The drawing under review shows one solid part. Ordinate dimensions are in mm from its lowest x, y, z. A direction names the side the tool comes from. Round coordinates to 2 decimals unless told otherwise and drop trailing zeros. Order: outer loops, then holes, each group sorted by start corner. A loop starts at its lowest first (then second) coordinate and runs counter-clockwise, first axis right, second up. Notation, with made-up numbers: (-14.75, -18) -> (2.25, -18) arc R27 cw to (2.25, 7) -> close; hole circle Ø11 at (-0.5, 12.5). An arc over 180 degrees is marked (long way). Return JSON: item names as keys, results as strings. Group by question number.
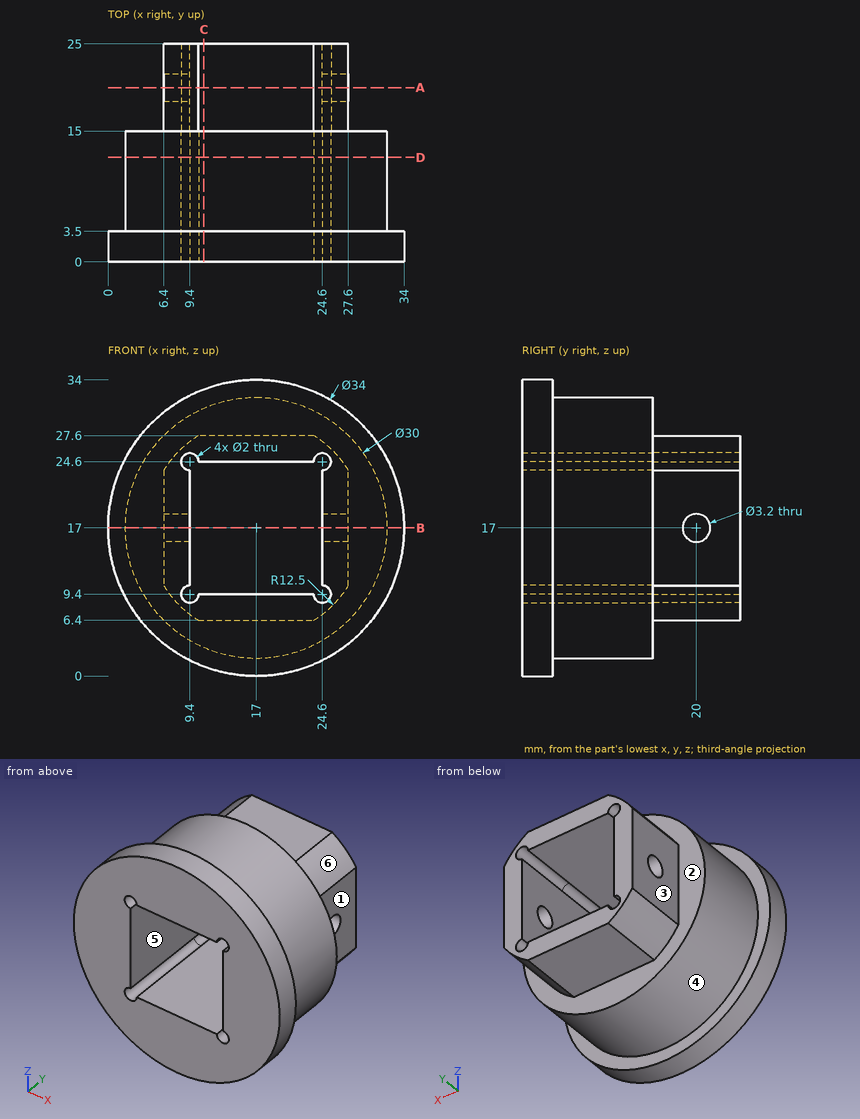
Item 1: Insertion check: pin 1 Ø5 at (y, z) = (18.5, 16) entering from -X; pin 2 Ø14.5 at (x, y) = (14, 16) entering from -Z; pin 3 Ø5 at (y, z) = (20, 17) entering from +X; pin 4 Ø8 at (x, z) = (26.5, 6.5) entering from -Y. Each pin has a flat end and moves straight along its axis. Give the tip position at first contact, or say it passes through.
Item 2: Consider section B-B on z = 17. State the section outline as (x, y) points, plus the area to 3 significant figures.
Item 3: Consider section A-A on y = 20. State the section outline as (x, z) points.
Item 4: Wall thickness on line 1 along X through (y, z) = (15.5, 19); line 2 along Y through (x, z) = (7.05, 17): over which ranges is each line inside the solid? List them lowest first.
Item 5: Consider section D-D on y = 12. State the section outline as (x, z) points, plus the area to 3 significant figures.
Item 6: Consider section C-C on x = 11. State the section outline as (y, z) points, plus the area to 3 significant figures.
Item 7: The part is to be moulded in two halves that separate along X. For the marked faces 4, 5 and 6, say which applies: +X half, -X half, draft (parallel to the pull), parting line (faces both ways), or undercut.
Item 8: For the marked faces 1, 2 and 3, list the 3-axis set-ups (+Z, -Z, +X, -X, +Y, -Y) from which the entire face can be reached by the end or side of a thin tool; tool diameter is ignored.
Values:
{
 "1": {"pin 1": "x = 6.4", "pin 2": "z = 2", "pin 3": "x = 27.6", "pin 4": "y = 0"},
 "2": {"outline": "(0, 0) -> (9.4, 0) -> (9.4, 18.4) -> (6.4, 18.4) -> (6.4, 15) -> (2, 15) -> (2, 3.5) -> (0, 3.5) -> close; (6.4, 21.6) -> (9.4, 21.6) -> (9.4, 25) -> (6.4, 25) -> close; (24.6, 0) -> (34, 0) -> (34, 3.5) -> (32, 3.5) -> (32, 15) -> (27.6, 15) -> (27.6, 18.4) -> (24.6, 18.4) -> close; (24.6, 21.6) -> (27.6, 21.6) -> (27.6, 25) -> (24.6, 25) -> close", "area": "277 mm^2"},
 "3": {"outline": "(6.4, 10.38) arc R12.5 ccw to (10.38, 6.4) -> (23.62, 6.4) arc R12.5 ccw to (27.6, 10.38) -> (27.6, 15.4) -> (24.6, 15.4) -> (24.6, 10.4) arc R1 cw (long way) to (23.6, 9.4) -> (10.4, 9.4) arc R1 cw (long way) to (9.4, 10.4) -> (9.4, 15.4) -> (6.4, 15.4) -> close; (6.4, 18.6) -> (9.4, 18.6) -> (9.4, 23.6) arc R1 cw (long way) to (10.4, 24.6) -> (23.6, 24.6) arc R1 cw (long way) to (24.6, 23.6) -> (24.6, 18.6) -> (27.6, 18.6) -> (27.6, 23.62) arc R12.5 ccw to (23.62, 27.6) -> (10.38, 27.6) arc R12.5 ccw to (6.4, 23.62) -> close"},
 "4": {"line 1": "6.4 to 9.4, 24.6 to 27.6", "line 2": "0 to 18.4, 21.6 to 25"},
 "5": {"outline": "circle Ø30 at (17, 17); hole (9.4, 10.4) arc R1 ccw (long way) to (10.4, 9.4) -> (23.6, 9.4) arc R1 ccw (long way) to (24.6, 10.4) -> (24.6, 23.6) arc R1 ccw (long way) to (23.6, 24.6) -> (10.4, 24.6) arc R1 ccw (long way) to (9.4, 23.6) -> close", "area": "466 mm^2"},
 "6": {"outline": "(0, 1.09) -> (3.5, 1.09) -> (3.5, 3.25) -> (15, 3.25) -> (15, 6.4) -> (25, 6.4) -> (25, 9.4) -> (0, 9.4) -> close; (0, 24.6) -> (25, 24.6) -> (25, 27.6) -> (15, 27.6) -> (15, 30.75) -> (3.5, 30.75) -> (3.5, 32.91) -> (0, 32.91) -> close", "area": "260 mm^2"},
 "7": {"face 4": "parting line", "face 5": "undercut", "face 6": "+X half"},
 "8": {"face 1": "+Z, -Z, +X, +Y", "face 2": "+Y", "face 3": "+Z, -Z, -X, +Y"}
}
